Part model, mm, in its own coordinate system. Give positions to 0.01 mm unless a question says otherwise; leave off trailing zeros. Write each loop counter-clockwise with the first axis right and the second up, starting at its lowest first coordinate (ties: lowest second). Pieces come first, ordered by that corner, then holes.
from build123d import *

# Parameters (mm, degrees)
BOSS_EXTRUDE1_DEPTH     = 8.3
SKETCH2_R               = 1.25
CUT_EXTRUDE1_DEPTH      = 3.700074126
CUT_EXTRUDE1_DEPTH_BACK = 1.323830371


with BuildPart() as part:
    # Sketch1 → Boss-Extrude1 (new body)
    with BuildSketch(Plane(origin=(0, 0, 0), x_dir=(1, 0, 0), z_dir=(0, 1, 0))):
        with BuildLine():
            Line((-17.5, 0.139549674), (-17.5, -1.870543406))
            ThreePointArc((-17.5, -1.870543406), (0.004776494, -2.697812194), (17.5, -1.688491505))
            Line((17.5, -1.688491505), (17.5, 0.323830371))
            ThreePointArc((17.5, 0.323830371), (0.004893833, -0.697784194), (-17.5, 0.139549674))
        make_face()
    extrude(amount=BOSS_EXTRUDE1_DEPTH)

    # Sketch2 → Cut-Extrude1 (cut, two sides)
    with BuildSketch(Plane.XY) as cut_extrude1_sk:
        with Locations((7.5, 4.15)):
            Circle(SKETCH2_R)
        with Locations((-7.5, 4.15)):
            Circle(SKETCH2_R)
    extrude(amount=CUT_EXTRUDE1_DEPTH, mode=Mode.SUBTRACT)
    extrude(cut_extrude1_sk.sketch, amount=-CUT_EXTRUDE1_DEPTH_BACK, mode=Mode.SUBTRACT)


solid = part.part
1) Saw through at A-A (x = 7.5). Write the cut outline in (y, z), and give its area (3 significant figures).
Check result:
outline: (0, 0.49) - (2.9, 0.49) - (2.9, 2.49) - (0, 2.49) - close; (5.4, 0.49) - (8.3, 0.49) - (8.3, 2.49) - (5.4, 2.49) - close
area: 11.6 mm2
2) Flat gauge pins, fed straight in: P1, Ø4, axis at x = -7.5, y = 4.15, coming from the -Z side; P2, Ø3, axis at x = 7.5, y = 4.15, coming from the +Z side; P3, Ø1, axis at y = 7, z = 2, coming from the -X side. Where does each tip first touch, or does it go through?
Check result:
P1: stops at z = 0.47
P2: stops at z = 2.56
P3: stops at x = -17.5
3) Drill centre lines: L1, parallel to X at y = 4.15, z = 0.95; L2, parallel to Y at x = -7.5, z = 1.3; L3, parallel to Z at x = 5.5, y = 3.75. Where is each one in solid material? Low to high.
Check result:
L1: x = -17.5 to -8.75, -6.25 to 6.25, 8.75 to 17.5
L2: y = 0 to 2.9, 5.4 to 8.3
L3: z = 0.58 to 2.58
4) Saw through at B-B (y = 4.15). Write the cut outline in (x, z).
Check result:
outline: (-17.5, -0.14) arc R165.21 cw to (-8.75, 0.51) - (-8.75, 2.51) arc R167.21 ccw to (-17.5, 1.87) - close; (-6.25, 0.61) arc R165.21 cw to (6.25, 0.55) - (6.25, 2.55) arc R167.21 ccw to (-6.25, 2.61) - close; (8.75, 0.42) arc R165.21 cw to (17.5, -0.32) - (17.5, 1.69) arc R167.21 ccw to (8.75, 2.42) - close
5) Mould opens along Y. For faces 1 (the flat face through (-17.5, 4, 1)), 2 (the flat face through (0, 0, 2)), 3 (the cylindrical face through (8.7, 4.5, 1.5)) say: +Y half, -Y half, draft (parallel to the pull), parting line (faces both ways), or undercut.
Check result:
face 1: draft
face 2: -Y half
face 3: undercut
6) Saw through at C-C (z = 1.25). Write the cut outline in (x, y).
Check result:
outline: (-17.5, 0) - (17.5, 0) - (17.5, 8.3) - (-17.5, 8.3) - close; hole circle Ø2.5 at (-7.5, 4.15); hole circle Ø2.5 at (7.5, 4.15)
7) Saw through at D-D (y = 7.5). Write the cut outline in (x, z).
Check result:
outline: (-17.5, -0.14) arc R165.21 cw to (17.5, -0.32) - (17.5, 1.69) arc R167.21 ccw to (-17.5, 1.87) - close
